```python
from build123d import *

# Parameters (mm, degrees)
ESBO_O1_W                = 60
ESBO_O1_H                = 140
RESSALTO_EXTRUS_O1_DEPTH = 15
FILETE1_R                = 2
CASCA1_T                 = 3
RESSALTO_EXTRUS_O2_START = 2.5
RESSALTO_EXTRUS_O2_DEPTH = 2.5
CORTE_EXTRUS_O1_REACH    = 101.956
ESBO_O4_W                = 7
ESBO_O4_H                = 5
CORTE_EXTRUS_O2_REACH    = 152.703
ESBO_O5_W                = 7
ESBO_O5_H                = 5
CORTE_EXTRUS_O3_REACH    = 101.956
ESBO_O6_W                = 7
ESBO_O6_H                = 5
CORTE_EXTRUS_O4_REACH    = 152.703
ESBO_O7_W                = 7
ESBO_O7_H                = 5


with BuildPart() as part:
    # Esboço1 → Ressalto-extrusão1 (new body)
    with BuildSketch(Plane(origin=(0, 0, 0), x_dir=(1, 0, 0), z_dir=(0, 1, 0))):
        Rectangle(ESBO_O1_W, ESBO_O1_H)
    extrude(amount=RESSALTO_EXTRUS_O1_DEPTH)

    # Filete1
    filete1_edges = [part.edges().sort_by_distance(p)[0] for p in [
        (0, 0, -70),
        (30, 0, 0),
        (0, 0, 70),
        (-30, 0, 0),
        (-30, 7.5, -70),
        (30, 7.5, -70),
        (30, 7.5, 70),
        (-30, 7.5, 70),
    ]]
    fillet(filete1_edges, radius=FILETE1_R)

    # Casca1
    casca1_openings = [part.faces().sort_by_distance(p)[0] for p in [
        (0, 15, 0),
    ]]
    offset(amount=CASCA1_T, openings=casca1_openings, kind=Kind.INTERSECTION)

    # Esboço3 → Ressalto-extrusão2 (add)
    with BuildSketch(Plane(origin=(0, 15, 0), x_dir=(1, 0, 0), z_dir=(0, 1, 0)).offset(RESSALTO_EXTRUS_O2_START)):
        with BuildLine():
            Line((28, 73), (-28, 73))
            ThreePointArc((-28, 73), (-31.535533906, 71.535533906), (-33, 68))
            Line((-33, 68), (-33, -68))
            ThreePointArc((-33, -68), (-31.535533906, -71.535533906), (-28, -73))
            Line((-28, -73), (28, -73))
            ThreePointArc((28, -73), (31.535533906, -71.535533906), (33, -68))
            Line((33, -68), (33, 68))
            ThreePointArc((33, 68), (31.535533906, 71.535533906), (28, 73))
        make_face()
        with BuildLine():
            Line((-31.8, 68), (-31.8, -68))
            ThreePointArc((-31.8, -68), (-30.687005769, -70.687005769), (-28, -71.8))
            Line((-28, -71.8), (28, -71.8))
            ThreePointArc((28, -71.8), (30.687005769, -70.687005769), (31.8, -68))
            Line((31.8, -68), (31.8, 68))
            ThreePointArc((31.8, 68), (30.687005769, 70.687005769), (28, 71.8))
            Line((28, 71.8), (-28, 71.8))
            ThreePointArc((-28, 71.8), (-30.687005769, 70.687005769), (-31.8, 68))
        make_face(mode=Mode.SUBTRACT)
    extrude(amount=-RESSALTO_EXTRUS_O2_DEPTH)

    # Esboço4 → Corte-extrusão1 (cut, up to next)
    with BuildSketch(Plane.ZY.offset(33), mode=Mode.PRIVATE) as corte_extrus_o1_sk1:
        with Locations((-57, 8.75)):
            Rectangle(ESBO_O4_W, ESBO_O4_H)
    corte_extrus_o1_tool1 = extrude(corte_extrus_o1_sk1.sketch, amount=-CORTE_EXTRUS_O1_REACH, mode=Mode.PRIVATE) & part.part
    add(corte_extrus_o1_tool1.solids().sort_by_distance((-33, 8.75, -57))[0], mode=Mode.SUBTRACT)

    # Esboço5 → Corte-extrusão2 (cut, up to next)
    with BuildSketch(Plane(origin=(0, 0, -73), x_dir=(-1, 0, 0), z_dir=(0, 0, -1)), mode=Mode.PRIVATE) as corte_extrus_o2_sk1:
        with Locations((15, 8.75)):
            Rectangle(ESBO_O5_W, ESBO_O5_H)
    corte_extrus_o2_tool1 = extrude(corte_extrus_o2_sk1.sketch, amount=-CORTE_EXTRUS_O2_REACH, mode=Mode.PRIVATE) & part.part
    add(corte_extrus_o2_tool1.solids().sort_by_distance((-15, 8.75, -73))[0], mode=Mode.SUBTRACT)

    # Esboço6 → Corte-extrusão3 (cut, up to next)
    with BuildSketch(Plane(origin=(33, 0, 0), x_dir=(0, 0, -1), z_dir=(1, 0, 0)), mode=Mode.PRIVATE) as corte_extrus_o3_sk1:
        with Locations((2, 8.75)):
            Rectangle(ESBO_O6_W, ESBO_O6_H)
    corte_extrus_o3_tool1 = extrude(corte_extrus_o3_sk1.sketch, amount=-CORTE_EXTRUS_O3_REACH, mode=Mode.PRIVATE) & part.part
    add(corte_extrus_o3_tool1.solids().sort_by_distance((33, 8.75, -2))[0], mode=Mode.SUBTRACT)

    # Esboço7 → Corte-extrusão4 (cut, up to next)
    with BuildSketch(Plane.XY.offset(73), mode=Mode.PRIVATE) as corte_extrus_o4_sk1:
        with Locations((0, 8.75)):
            Rectangle(ESBO_O7_W, ESBO_O7_H)
    corte_extrus_o4_tool1 = extrude(corte_extrus_o4_sk1.sketch, amount=-CORTE_EXTRUS_O4_REACH, mode=Mode.PRIVATE) & part.part
    add(corte_extrus_o4_tool1.solids().sort_by_distance((0, 8.75, 73))[0], mode=Mode.SUBTRACT)


solid = part.part
```
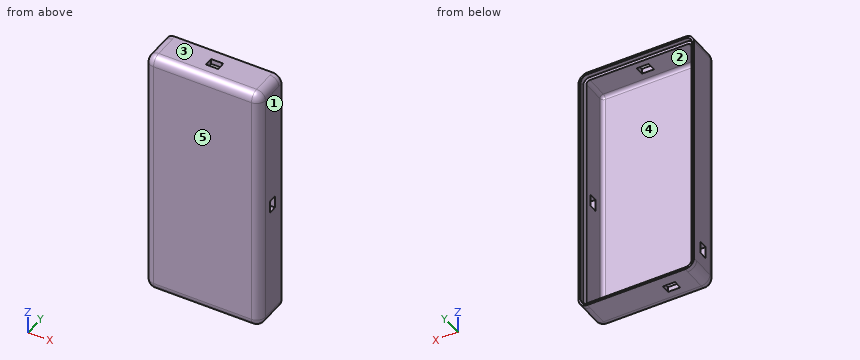
Work out the finished part from the listing and answer in its coordinate system (mm). Face numbers are marked on the shaded views. A direction names the side the tool comes from. Give positions to 0.01 mm unless a question says otherwise; leave off trailing zeros. Loops run counter-clockwise (first coordinate to the right, second up) from the corner with the lowest first, then second, coordinate; pieces in that order, holes last. Notation, with made-up numbers: M 88.5,1 L 115.5,1 A19 cw 115.5,7 Z; hole C 64.25,43 d8. An arc over 180 degrees is marked long. One line per item, written item: value. Start each with the question number.
1. Find section B-B (x = 0). Give the vertices of the cut face in (y, z).
2. Determine the mould class of the marked faces 1, 2 and 3 for opening direction Z: released by +Z, released by -Z, zero draft, split by the parting line, or undercut.
3. Find section C-C (z = 12). Give the vertices of the cut face in (x, y), and give its area (3 significant figures).
4. Each of these flat-tipped pins is pushed along its axis until it touches: P1, Ø1.5, axis at x = -31.5, y = 8.5, coming from the -Z side; P2, Ø1.5, axis at x = -32, y = 9, coming from the +Z side; P3, Ø5, axis at x = 3, z = 30, coming from the +Y side. Where does it stop, or does it pass through?
5. Which of the six approach directions +Z, -Z, +X, -X, +Y, -Y give full straight-line access (tool end or side, diameter ignored) to the marked faces 4 and 5?
6. Find section D-D (x = -23.5). Give the vertices of the cut face in (y, z), and give its area (3 significant figures).
7. Find section A-A (y = 8.75). State how many separate pieces and enclosed holes the cut face has, and give its area (3 significant figures).
8. Find the intervals of material crossed by probe 1 along Z at (x, y) = (13.5, 2.5); probe 2 along X at (y, z) = (13.5, 39); probe 3 along Y at (x, z) = (-3.5, -17), in increasing order.
Reported:
1. outline: M -3,-68 A5 ccw 2,-73 L 17.5,-73 L 17.5,-71.8 L 15,-71.8 L 15,-70 L 2,-70 A2 cw 0,-68 L 0,68 A2 cw 2,70 L 6.25,70 L 6.25,73 L 2,73 A5 ccw -3,68 Z; M 11.25,70 L 15,70 L 15,71.8 L 17.5,71.8 L 17.5,73 L 11.25,73 Z
2. face 1: zero draft
2. face 2: undercut
2. face 3: released by +Z
3. outline: M -33,2 A5 ccw -28,-3 L 28,-3 A5 ccw 33,2 L 33,17.5 L 31.8,17.5 L 31.8,15 L 30,15 L 30,2 A2 cw 28,0 L -28,0 A2 cw -30,2 L -30,15 L -31.8,15 L -31.8,17.5 L -33,17.5 Z
3. area: 285 mm²
4. P1: stops at z = -72.18
4. P2: stops at z = 71.8
4. P3: stops at y = 0
5. face 4: +Y
5. face 5: +Z, -Z, +X, -X, -Y
6. outline: M -3,-68 A5 ccw 2,-73 L 17.5,-73 L 17.5,-71.8 L 15,-71.8 L 15,-70 L 2,-70 A2 cw 0,-68 L 0,68 A2 cw 2,70 L 15,70 L 15,71.8 L 17.5,71.8 L 17.5,73 L 2,73 A5 ccw -3,68 Z
6. area: 525 mm²
7. separate pieces: 4
7. enclosed holes: 0
7. area: 1,130 mm²
8. probe 1: z = -73 to -70, 70 to 73
8. probe 2: x = -33 to -30, 30 to 33
8. probe 3: y = -3 to 0
